The drawing under review shows one solid part. Ordinate dimensions are in mm from its lowest x, y, z. Coordinates: 2 decimals unless noted, no trailing zeros. Write each loop counter-clockwise with the first axis right and the second up, starting at its lowest first coordinate (ties: lowest second). Pieces come first, ordered by that corner, then holes.
1) Add section A-A, the plane z = 12.7. State the section outline as (x, y) points (1 decimal).
2) For line 1 (X direction, y = 0.85, z = 12.7); line 2 (X direction, y = 1.25, z = 11.75); line 3 (X direction, y = 1.3, z = 24), list the stretches that pass through material, from the lowest coordinate up.
3) Mouldability with a two-part tool opening along Z and no side actions: class the marked faces 1, 2 and 3 as released by +Z, released by -Z, zero draft, split by the parting line, or undercut.
4) Add section C-C, the plane x = 12.7. State the section outline as (y, z) points (1 decimal).
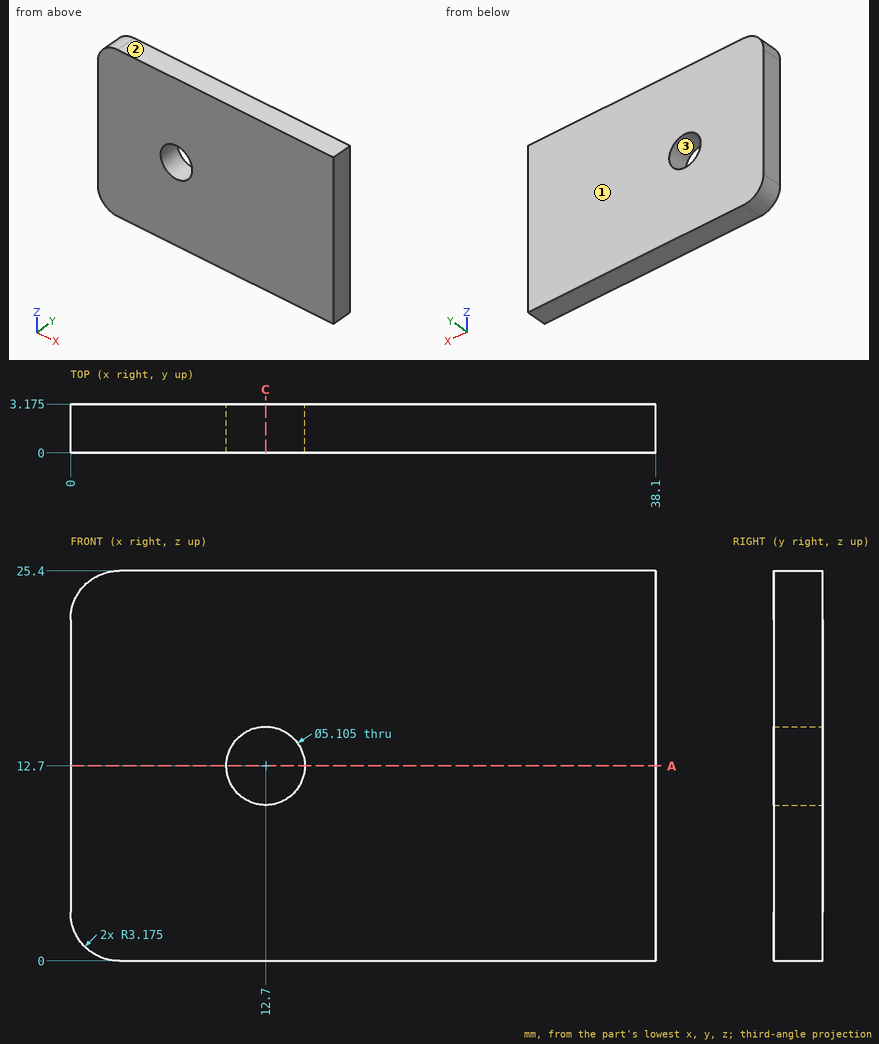
Geometry results:
1. outline: (0, 0) - (10.1, 0) - (10.1, 3.2) - (0, 3.2) - close; (15.3, 0) - (38.1, 0) - (38.1, 3.2) - (15.3, 3.2) - close
2. line 1: x = 0 to 10.15, 15.25 to 38.1
2. line 2: x = 0 to 10.33, 15.07 to 38.1
2. line 3: x = 0.54 to 38.1
3. face 1: zero draft
3. face 2: released by +Z
3. face 3: undercut
4. outline: (0, 0) - (3.2, 0) - (3.2, 10.1) - (0, 10.1) - close; (0, 15.3) - (3.2, 15.3) - (3.2, 25.4) - (0, 25.4) - close
